from build123d import *

# Parameters (mm, degrees)
SKETCH_W        = 60
SKETCH_H        = 25
PAD_DEPTH       = 7
SKETCH002_R     = 3
POCKET_DEPTH    = 7.001
SKETCH003_W     = 2.9
SKETCH003_H     = 15
SKETCH003_W_2   = 3
PAD001_DEPTH    = 17
SKETCH005_R     = 6
PAD002_DEPTH    = 3
POCKET001_DEPTH = 3
SKETCH007_R     = 2.6
POCKET002_DEPTH = 37.551
FILLET_R        = 7
CHAMFER_SIZE    = 6
CHAMFER001_SIZE = 1


with BuildPart() as part:
    # Sketch → Pad (new body)
    with BuildSketch(Plane.XY):
        Rectangle(SKETCH_W, SKETCH_H)
    extrude(amount=PAD_DEPTH)

    # Sketch002 (on Face6 of Pad) → Pocket (cut, through all)
    with BuildSketch(Plane.XY.offset(7)):
        Circle(SKETCH002_R)
    extrude(amount=-POCKET_DEPTH, mode=Mode.SUBTRACT)

    # Sketch003 (on Face6 of Pocket) → Pad001 (join)
    with BuildSketch(Plane.XZ.offset(12.5)):
        with Locations((0, 7.5)):
            Rectangle(SKETCH003_W, SKETCH003_H)
        with Locations((6.05, 7.5)):
            Rectangle(SKETCH003_W_2, SKETCH003_H)
        with Locations((-6.05, 7.5)):
            Rectangle(SKETCH003_W_2, SKETCH003_H)
    extrude(amount=PAD001_DEPTH)

    # Sketch005 (on Face18 of Pad001) → Pad002 (join)
    with BuildSketch(Plane.YZ.offset(7.55)):
        with Locations((-22, 7.5)):
            Circle(SKETCH005_R)
    extrude(amount=PAD002_DEPTH)

    # Sketch006 (on Face30 of Pad002) → Pocket001 (cut)
    with BuildSketch(Plane.YZ.offset(10.55)):
        Polygon((-17.925, 9.852702), (-22, 12.205405), (-26.075, 9.852702), (-26.075, 5.147298), (-22, 2.794595), (-17.925, 5.147298), align=None)
    extrude(amount=-POCKET001_DEPTH, mode=Mode.SUBTRACT)

    # Sketch007 (on Face37 of Pocket001) → Pocket002 (cut, through all)
    with BuildSketch(Plane.YZ.offset(7.55)):
        with Locations((-22, 7.5)):
            Circle(SKETCH007_R)
    extrude(amount=-POCKET002_DEPTH, mode=Mode.SUBTRACT)

    # Fillet
    fillet_edges = [part.edges().sort_by_distance(p)[0] for p in [
        (0, -29.5, 15),
        (-6.05, -29.5, 15),
        (6.05, -29.5, 15),
        (6.05, -29.5, 0),
        (0, -29.5, 0),
        (-6.05, -29.5, 0),
    ]]
    fillet(fillet_edges, radius=FILLET_R)

    # Chamfer
    chamfer_edges = [part.edges().sort_by_distance(p)[0] for p in [
        (6.05, -12.5, 7),
        (0, -12.5, 7),
        (-6.05, -12.5, 7),
    ]]
    chamfer(chamfer_edges, length=CHAMFER_SIZE)

    # Chamfer001
    chamfer001_edges = [part.edges().sort_by_distance(p)[0] for p in [
        (6.05, -12.5, 15),
        (0, -12.5, 15),
        (-6.05, -12.5, 15),
    ]]
    chamfer(chamfer001_edges, length=CHAMFER001_SIZE)


solid = part.part
For this review, take the finished solid that the model builds, in its own axes (mm). A direction names the side the tool comes from. Round coordinates to 2 decimals unless told otherwise and drop trailing zeros. Write each loop counter-clockwise with the first axis right and the second up, starting at its lowest first coordinate (ties: lowest second). Pieces come first, ordered by that corner, then holes. Notation, with made-up numbers: (58.25, 19) - (95.25, 19) arc R27 cw to (95.25, 57) - close; hole circle Ø2 at (89, 46.25). An arc over 180 degrees is marked (long way). Use a Markdown table: item, result.
Q1. We need section D-D (y = -20.5). State how many separate pieces and enclosed holes the cut face has, plus the area to 3 significant figures.
Derived:
| item | result |
|---|---|
| separate pieces | 6 |
| enclosed holes | 0 |
| area | 108 mm2 |
Q2. Clearance check with flat-ended pins moving along their axes: pin 1 (0.8 mm diameter, centred on x = 0, z = 13.5, fed in from +Y); pin 2 (3.5 mm diameter, centred on x = 3.5, z = 3, fed in from -Y); pin 3 (10 mm diameter, centred on x = -17, y = -21, fed in from -Z); pin 4 (3.5 mm diameter, centred on y = -19, z = 10, fed in from +X). State where each tip first meets the part, or that it passes through.
Derived:
| item | result |
|---|---|
| pin 1 | stops at y = -12.5 |
| pin 2 | stops at y = -29 |
| pin 3 | passes through |
| pin 4 | stops at x = 10.55 |
Q3. The part is to be moulded in two halves that separate along Y. For faces 4 (the flat face through (9.071, -19.991, 3.954)), 5 (the flat face through (-6.1, -9.5, 10)), 6 (the cylindrical face through (-6, -27.5, 12.9)), 7 (the flat face through (30, 0, 3)), say which applies: pulls with the +Y half, pulls with the -Y half, needs draft (parallel to the pull), parting line crosses it, or undercut.
Derived:
| item | result |
|---|---|
| face 4 | undercut |
| face 5 | pulls with the +Y half |
| face 6 | pulls with the -Y half |
| face 7 | needs draft |
Q4. We need section A-A (x = 0). Give the boundary of the cut face in (y, z), plus the area to 3 significant figures.
Derived:
| item | result |
|---|---|
| outline | (-29.5, 7) arc R7 ccw to (-22.5, 0) - (-3, 0) - (-3, 7) - (-6.5, 7) - (-12.5, 13) - (-12.5, 14) - (-13.5, 15) - (-22.5, 15) arc R7 ccw to (-29.5, 8) - close; (3, 0) - (12.5, 0) - (12.5, 7) - (3, 7) - close; hole circle Ø5.2 at (-22, 7.5) |
| area | 363 mm2 |
Q5. We need section C-C (y = -11.5). Give the boundary of the cut face in (x, z).
Derived:
| item | result |
|---|---|
| outline | (-30, 0) - (30, 0) - (30, 7) - (7.55, 7) - (7.55, 12) - (4.55, 12) - (4.55, 7) - (1.45, 7) - (1.45, 12) - (-1.45, 12) - (-1.45, 7) - (-4.55, 7) - (-4.55, 12) - (-7.55, 12) - (-7.55, 7) - (-30, 7) - close |
Q6. Wall thickness on line 1 along X through (y, z) = (-9, 8); line 2 along Z through (x, y) = (0.5, -22); line 3 along Z through (x, y) = (-20, -5): over which ranges is each line inside the solid? List them lowest first.
Derived:
| item | result |
|---|---|
| line 1 | x = -7.55 to -4.55, -1.45 to 1.45, 4.55 to 7.55 |
| line 2 | z = 0 to 4.9, 10.1 to 15 |
| line 3 | z = 0 to 7 |
Q7. Machinability: for faces 1 (the flat face through (6, -18, 15)), 2 (the flat face through (9, -26.075, 8)), 3 (the flat face through (3, -12.5, 3)), which of the approach directions +Z, -Z, +X, -X, +Y, -Y give a long, thin tool a straight path to every point of the face, cutting with its end or side? Answer none if there is none.
Derived:
| item | result |
|---|---|
| face 1 | +Z, +X, -X, +Y, -Y |
| face 2 | +X |
| face 3 | +Z, -Z, -Y |
Q8. We need section B-B (y = 0). Give the boundary of the cut face in (x, z), plus the area to 3 significant figures.
Derived:
| item | result |
|---|---|
| outline | (-30, 0) - (-3, 0) - (-3, 7) - (-30, 7) - close; (3, 0) - (30, 0) - (30, 7) - (3, 7) - close |
| area | 378 mm2 |
